Geometry check sheet. Reference: the model listing, model coordinates, mm. A direction names the side the tool comes from. Coordinates: 2 decimals unless noted, no trailing zeros. Write each loop counter-clockwise with the first axis right and the second up, starting at its lowest first coordinate (ties: lowest second). Pieces come first, ordered by that corner, then holes. Notation, with made-up numbers: M 56,13.25 L 95,13.25 A18 ccw 95,36.25 Z; hole C -25.5,-16.75 d9. An arc over 180 degrees is marked long. Answer as a JSON object with one key per item and string values. Group by question number.
```python
from build123d import *

# Parameters (mm, degrees)
TABAN_FLAN_1_DEPTH           = 9
KENAR_FLAN_1_STRIP_CUT_DEPTH = 18
KENAR_FLAN_1_DEPTH           = 18
KENAR_FLAN_1_START           = 0.5
KENAR_FLAN_1_FLAT_DEPTH      = 0.5
DIKI_1_START                 = -9
DIKI_1_DEPTH                 = 18
IZIM24_W                     = 18
IZIM24_H                     = 7
SEKME3_DEPTH                 = 0.5
KENAR_FLAN_2_STRIP_CUT_DEPTH = 18
KENAR_FLAN_2_DEPTH           = 18
KENAR_FLAN_2_START           = 0.5
KENAR_FLAN_2_FLAT_DEPTH      = 0.5
KES_EKSTR_ZYON1_REACH        = 24.729
KES_EKSTR_ZYON2_REACH        = 24.841


# Read off the part's stored shape, not the designer's step: Dikiş1
# Sheet-metal steps are written as plain solids
with BuildPart() as part:
    # Çizim1 → Taban-Flanş1 (new, symmetric)
    with BuildSketch(Plane.XY):
        Polygon((0, 0), (1.255616527, 17.956152905), (1.754398553, 17.921274668), (0.498782025, -0.034878237), align=None)
    extrude(amount=TABAN_FLAN_1_DEPTH, both=True)

    # Kenar-Flanş1 strip (across the edge) → Kenar-Flanş1 strip cut (cut)
    with BuildSketch(Plane(origin=(0.498782025, -0.034878237, 9), x_dir=(0.9762960071199348, 0.2164396139380966, 0), z_dir=(0, 0, -1))):
        Polygon((-6.3159448, 19.561804043), (-0.067607216, -1.532230124), (0.411802651, -1.390222452), (-5.836534932, 19.703811715), align=None)
    extrude(amount=KENAR_FLAN_1_STRIP_CUT_DEPTH, mode=Mode.SUBTRACT)

    # Kenar-Flanş1 bend section (across the edge) → Kenar-Flanş1 (add)
    with BuildSketch(Plane(origin=(0.498782025, -0.034878237, 9), x_dir=(0.9762960071199348, 0.2164396139380966, 0), z_dir=(0, 0, -1))):
        with BuildLine():
            Line((-0.5, 1.449930995), (0, 1.449930995))
            ThreePointArc((0, 1.449930995), (0.103486132, 0.015004775), (0.411802651, -1.390222452))
            Line((0.411802651, -1.390222452), (-0.067607216, -1.532230124))
            ThreePointArc((-0.067607216, -1.532230124), (-0.391339562, -0.056741536), (-0.5, 1.449930995))
        make_face()
    extrude(amount=KENAR_FLAN_1_DEPTH)

    # Kenar-Flanş1 profile (on flange) → Kenar-Flanş1 flat (add)
    with BuildSketch(Plane(origin=(0.498782025, -0.034878237, 0), x_dir=(0, 0, -1), z_dir=(-0.9762960071199348, -0.2164396139380966, 0)).offset(KENAR_FLAN_1_START)):
        with BuildLine():
            ThreePointArc((9, 3.9408211), (0, 5.9408211), (-9, 3.9408211))
            Line((-9, 3.9408211), (-9, 1.449930995))
            Line((-9, 1.449930995), (9, 1.449930995))
            Line((9, 1.449930995), (9, 3.9408211))
        make_face()
    extrude(amount=-KENAR_FLAN_1_FLAT_DEPTH)

    # Dikiş1 outline → Dikiş1 (add)
    with BuildSketch(Plane.XY.offset(DIKI_1_START)):
        with BuildLine():
            Line((-0.542336916, -0.13733327), (-0.047828985, -0.063428564))
            Line((-0.047828985, -0.063428564), (-2.7175433, 17.80004703))
            ThreePointArc((-2.7175433, 17.80004703), (-0.818031205, 20.094123925), (1.255616527, 17.956152905))
            Line((1.255616527, 17.956152905), (1.754398553, 17.921274668))
            ThreePointArc((1.754398553, 17.921274668), (-0.837661113, 20.593738443), (-3.212051232, 17.726142324))
            Line((-3.212051232, 17.726142324), (-0.542336916, -0.13733327))
        make_face()
    extrude(amount=DIKI_1_DEPTH)

    # Çizim24 → Sekme3 (add)
    with BuildSketch(Plane(origin=(-0.550564326, -0.08228239, 0), x_dir=(0, 0, 1), z_dir=(-0.989015863361916, -0.1478094111296166, 0))):
        with Locations((0, -3.555662282)):
            Rectangle(IZIM24_W, IZIM24_H)
    extrude(amount=-SEKME3_DEPTH)

    # Kenar-Flanş2 strip (across the edge) → Kenar-Flanş2 strip cut (cut)
    with BuildSketch(Plane(origin=(0.492328961, -7.060444313, -9), x_dir=(-0.8788171126619707, 0.4771587602595987, 0), z_dir=(0, 0, 1))):
        Polygon((-6.614275583, 7.946620091), (0.607504695, -1.63700603), (1.00682245, -1.336098518), (-6.214957828, 8.247527602), align=None)
    extrude(amount=KENAR_FLAN_2_STRIP_CUT_DEPTH, mode=Mode.SUBTRACT)

    # Kenar-Flanş2 bend section (across the edge) → Kenar-Flanş2 (add)
    with BuildSketch(Plane(origin=(0.492328961, -7.060444313, -9), x_dir=(-0.8788171126619707, 0.4771587602595987, 0), z_dir=(0, 0, 1))):
        with BuildLine():
            Line((-0.5, 1.672976598), (0, 1.672976598))
            ThreePointArc((0, 1.672976598), (0.258381724, 0.086453315), (1.00682245, -1.336098518))
            Line((1.00682245, -1.336098518), (0.607504695, -1.63700603))
            ThreePointArc((0.607504695, -1.63700603), (-0.215780104, -0.072199013), (-0.5, 1.672976598))
        make_face()
    extrude(amount=KENAR_FLAN_2_DEPTH)

    # Kenar-Flanş2 profile (on flange) → Kenar-Flanş2 flat (add)
    with BuildSketch(Plane(origin=(0.492328961, -7.060444313, 0), x_dir=(0, 0, 1), z_dir=(0.8788171126619707, -0.4771587602595987, 0)).offset(KENAR_FLAN_2_START)):
        with BuildLine():
            ThreePointArc((9, 2.63270234), (0, 8.13270234), (-9, 2.63270234))
            Line((-9, 2.63270234), (-9, 1.672976598))
            Line((-9, 1.672976598), (9, 1.672976598))
            Line((9, 1.672976598), (9, 2.63270234))
        make_face()
    extrude(amount=-KENAR_FLAN_2_FLAT_DEPTH)

    # Çizim31 → Kes-Ekstrüzyon1 (cut, up to next)
    with BuildSketch(Plane(origin=(-0.550564326, -0.08228239, 0), x_dir=(0, 0, 1), z_dir=(-0.9890158633619159, -0.1478094111296166, 0)), mode=Mode.PRIVATE) as kes_ekstr_zyon1_sk1:
        with BuildLine():
            Line((-3.55, 10.956207356), (-3.55, 4.156207356))
            ThreePointArc((-3.55, 4.156207356), (0, 0.606207356), (3.55, 4.156207356))
            Line((3.55, 4.156207356), (3.55, 10.956207356))
            ThreePointArc((3.55, 10.956207356), (0, 14.506207356), (-3.55, 10.956207356))
        make_face()
    kes_ekstr_zyon1_tool1 = extrude(kes_ekstr_zyon1_sk1.sketch, amount=-KES_EKSTR_ZYON1_REACH, mode=Mode.PRIVATE) & part.part
    add(kes_ekstr_zyon1_tool1.solids().sort_by_distance((-1.667443, 7.390927, 0))[0], mode=Mode.SUBTRACT)

    # Çizim32 → Kes-Ekstrüzyon2 (cut, up to next)
    with BuildSketch(Plane(origin=(0.498782025, -0.034878237, 0), x_dir=(0, 0, -1), z_dir=(0.9975640502598243, -0.06975647374412548, 0)), mode=Mode.PRIVATE) as kes_ekstr_zyon2_sk1:
        with BuildLine():
            Line((1.7, 8.550531975), (1.7, 3.937201267))
            ThreePointArc((1.7, 3.937201267), (0, 2.237201267), (-1.7, 3.937201267))
            Line((-1.7, 3.937201267), (-1.7, 8.550531975))
            ThreePointArc((-1.7, 8.550531975), (0, 13.8), (1.7, 8.550531975))
        make_face()
    kes_ekstr_zyon2_tool1 = extrude(kes_ekstr_zyon2_sk1.sketch, amount=-KES_EKSTR_ZYON2_REACH, mode=Mode.PRIVATE) & part.part
    add(kes_ekstr_zyon2_tool1.solids().sort_by_distance((1.098249, 8.537894, 0))[0], mode=Mode.SUBTRACT)


solid = part.part
```
1) Section check A-A (y = 6). Record the cut outline in (x, z), then the cut area to 3 significant figures.
2) Set-up check for faces 5 (the flat face through (-1.4, 7.5, -3.55)), 6 (the flat face through (0.54, 7.75, -1.87)), 7 (the cylindrical face through (-2.45, 14.3, 0.08)): record each of +Z, -Z, +X, -X, +Y, -Y from which the full face is reachable in a straight line by a thin tool's end or side.
3) Material ranges on probe 1 along Z at (x, y) = (0.7, 6); probe 2 along Y at (x, z) = (-1.15, 1.5); probe 3 along Y at (x, z) = (-1.7, -0.25), recorded low to high. Write a range as [from, to].
4) Draft check along Z on faces 1 (the cylindrical face through (-3.16, -14.33, 0.16)), 2 (the flat face through (0.9, 8.2, -9)), 3 (the cylindrical face through (0.6, 0, 0.1)), 4 (the cylindrical face through (1.215, 13.747, 0.102)). Enter one of: +Z half, -Z half, draft (parallel to the pull), parting line (faces both ways), or undercut.
5) Section check C-C (z = -4.25). Record the cut outline in (x, y), then the cut area to 3 significant figures.
6) Section check B-B (z = 6.5). Record the cut outline in (x, y), then the cut area to 3 significant figures.
7) Go/stop test with flat-tipped pins: pin 1 Ø6 at (y, z) = (-4.5, -1.5) entering from -X; pin 2 Ø10 at (y, z) = (12.5, -5) entering from -X; pin 3 Ø4 at (y, z) = (4, -7) entering from +X. Record where each tip stops, or that it passes through.
8) Section check D-D (y = -8). Record the cut outline in (x, z), then the cut area to 3 significant figures.
Entries:
{
 "1": {"outline": "M -1.46,-9 L -0.95,-9 L -0.95,-3.55 L -1.46,-3.55 Z; M -1.46,3.55 L -0.95,3.55 L -0.95,9 L -1.46,9 Z; M 0.42,-9 L 0.92,-9 L 0.92,-1.7 L 0.42,-1.7 Z; M 0.42,1.7 L 0.92,1.7 L 0.92,9 L 0.42,9 Z", "area": "12.8 mm^2"},
 "2": {"face 5": "-X", "face 6": "+Z, -Z", "face 7": "none"},
 "3": {"probe 1": "[-9, -1.7], [1.7, 9]", "probe 2": "[-11.13, -10.09], [20.05, 20.56]", "probe 3": "[-12.15, -11.1], [19.85, 20.4]"},
 "4": {"face 1": "parting line", "face 2": "-Z half", "face 3": "draft", "face 4": "undercut"},
 "5": {"outline": "M -3.21,17.73 L 0.25,-5.41 A5 cw -0.31,-8.53 L -2.94,-13.38 L -2.5,-13.62 L 0.13,-8.77 A5.5 ccw 0.74,-5.33 L -2.72,17.8 A2 cw long 1.26,17.96 L 0.1,1.45 A10.5 ccw 0.32,-1.56 L 1.2,-5.52 L 1.69,-5.42 L 0.81,-1.45 A10 cw 0.6,1.41 L 1.75,17.92 A2.5 ccw long Z", "area": "31.7 mm^2"},
 "6": {"outline": "M -3.21,17.73 L 0.25,-5.41 A5 cw -0.31,-8.53 L -2.26,-12.13 L -1.82,-12.37 L 0.13,-8.77 A5.5 ccw 0.74,-5.33 L -2.72,17.8 A2 cw long 1.26,17.96 L 0.1,1.45 A10.5 ccw 0.32,-1.56 L 1.08,-4.95 L 1.56,-4.84 L 0.81,-1.45 A10 cw 0.6,1.41 L 1.75,17.92 A2.5 ccw long Z", "area": "30.7 mm^2"},
 "7": {"pin 1": "x = -0.34", "pin 2": "x = -3.18", "pin 3": "x = 0.92"},
 "8": {"outline": "M -0.06,-9 L 0.48,-9 L 0.48,9 L -0.06,9 Z", "area": "9.62 mm^2"}
}
